```python
from build123d import *

# Parameters (mm, degrees)
BOSS_EXTRUDE1_DEPTH  = 12.5
M5_CLEARANCE_HOLE1_D = 5.3
SKETCH4_W            = 1
SKETCH4_H            = 20
BOSS_EXTRUDE2_DEPTH  = 3


with BuildPart() as part:
    # Sketch1 → Boss-Extrude1 (new body, symmetric)
    with BuildSketch(Plane.XY):
        with BuildLine():
            Line((-15.2, 0), (-12.7, 0))
            ThreePointArc((-12.7, 0), (0, 12.7), (12.7, 0))
            Line((12.7, 0), (15.2, 0))
            Line((15.2, 0), (15.2, 5.2))
            ThreePointArc((15.2, 5.2), (12.271067812, 12.271067812), (5.2, 15.2))
            Line((5.2, 15.2), (-5.2, 15.2))
            ThreePointArc((-5.2, 15.2), (-12.271067812, 12.271067812), (-15.2, 5.2))
            Line((-15.2, 5.2), (-15.2, 0))
        make_face()
    extrude(amount=BOSS_EXTRUDE1_DEPTH, both=True)

    # M5 Clearance Hole1 (through all)
    with Locations(Plane(origin=(0, 15.2, 0), x_dir=(1, 0, 0), z_dir=(0, 1, 0))):
        with Locations((0, 0)):
            Hole(M5_CLEARANCE_HOLE1_D / 2)

    # Sketch4 → Boss-Extrude2 (add)
    with BuildSketch(Plane.XZ):
        with Locations((-13.95, 0)):
            Rectangle(SKETCH4_W, SKETCH4_H)
        with Locations((13.95, 0)):
            Rectangle(SKETCH4_W, SKETCH4_H)
    extrude(amount=BOSS_EXTRUDE2_DEPTH)


solid = part.part
```
CAD build for the part. Positions are in the model's coordinates, mm. A direction names the side the tool comes from. Round coordinates to 2 decimals unless told otherwise and drop trailing zeros. Order: outer loops, then holes, each group sorted by start corner. A loop starts at its lowest first (then second) coordinate and runs counter-clockwise, first axis right, second up. Notation, with made-up numbers: (51.25, 33) - (108.25, 33) arc R13 ccw to (108.25, 57) - close; hole circle Ø11 at (-37.5, 24). An arc over 180 degrees is marked (long way). Answer in a Markdown table with one row per item. Add a question column.
(1) Band-saw the part on D-D on y = 2.5. List the corners of the cut face in (x, z), and give its area (3 significant figures).
(2) Band-saw the part on A-A on x = 0. List the corners of the cut face in (y, z), and give its area (4 significant figures).
(3) Probe L1, parallel to Z at x = 0, y = 13.6; L2, parallel to X at y = -0.5, z = -6; L3, parallel to X at y = 3.5, z = 5.5. List the from-to ranges inside material, lowest first. Write a range as [from, to].
(4) Band-saw the part on C-C on z = -10.5. List the corners of the cut face in (x, y).
(5) Mould opens along X. For faces 1 (the face through (15.2, 3, 0)), 2 (the face through (-14, -1, -10)), 3 (the face through (13, 0, 0)) say: +X half, -X half, draft (parallel to the pull), parting line (faces both ways), or undercut.
(6) 3-axis set-ups, long thin cutter, end or side, ignore diameter. For faces 4 (the face through (14.45, -1, 0)), 5 (the face through (13.45, -1, 0)), 6 (the face through (14, -1, 10)): which of +Z, -Z, +X, -X, +Y, -Y reach the whole face in a straight line?
(7) Drop flat-ended pins along their axis: pin 1 Ø5 at (x, z) = (-6, -6.5) entering from -Y; pin 2 Ø1.1 at (x, y) = (14, -2) entering from -Z; pin 3 Ø0.9 at (y, z) = (-1, -4.5) entering from +X; pin 4 Ø3 at (x, z) = (0, 0) entering from -Y. Give the stop position or say it passes through.
(8) Band-saw the part on B-B on z = 0. List the corners of the cut face in (x, y), and give its area (3 significant figures).
Data:
| question | item | result |
|---|---|---|
| 1 | outline | (-15.2, -12.5) - (-12.45, -12.5) - (-12.45, 12.5) - (-15.2, 12.5) - close; (12.45, -12.5) - (15.2, -12.5) - (15.2, 12.5) - (12.45, 12.5) - close |
| 1 | area | 137 mm^2 |
| 2 | outline | (12.7, -12.5) - (15.2, -12.5) - (15.2, -2.65) - (12.7, -2.65) - close; (12.7, 2.65) - (15.2, 2.65) - (15.2, 12.5) - (12.7, 12.5) - close |
| 2 | area | 49.25 mm^2 |
| 3 | L1 | z = [-12.5, -2.65], [2.65, 12.5] |
| 3 | L2 | x = [-14.45, -13.45], [13.45, 14.45] |
| 3 | L3 | x = [-15.2, -12.21], [12.21, 15.2] |
| 4 | outline | (-15.2, 0) - (-12.7, 0) arc R12.7 cw to (12.7, 0) - (15.2, 0) - (15.2, 5.2) arc R10 ccw to (5.2, 15.2) - (-5.2, 15.2) arc R10 ccw to (-15.2, 5.2) - close |
| 5 | face 1 | +X half |
| 5 | face 2 | draft |
| 5 | face 3 | undercut |
| 6 | face 4 | +Z, -Z, +X, -Y |
| 6 | face 5 | +Z, -Z, -Y |
| 6 | face 6 | +Z, +X, -X, -Y |
| 7 | pin 1 | stops at y = 9.44 |
| 7 | pin 2 | stops at z = -10 |
| 7 | pin 3 | stops at x = 14.45 |
| 7 | pin 4 | passes through |
| 8 | outline | (-15.2, 0) - (-14.45, 0) - (-14.45, -3) - (-13.45, -3) - (-13.45, 0) - (-12.7, 0) arc R12.7 cw to (-2.65, 12.42) - (-2.65, 15.2) - (-5.2, 15.2) arc R10 ccw to (-15.2, 5.2) - close; (2.65, 12.42) arc R12.7 cw to (12.7, 0) - (13.45, 0) - (13.45, -3) - (14.45, -3) - (14.45, 0) - (15.2, 0) - (15.2, 5.2) arc R10 ccw to (5.2, 15.2) - (2.65, 15.2) - close |
| 8 | area | 158 mm^2 |
